from build123d import *

# Parameters (mm, degrees)
SKETCH1_W           = 37
SKETCH1_H           = 22
BOSS_EXTRUDE1_DEPTH = 10
SKETCH3_W           = 37
SKETCH3_H           = 22
BOSS_EXTRUDE2_DEPTH = 9
SKETCH5_W           = 5
SKETCH5_H           = 3
BOSS_EXTRUDE3_DEPTH = 5
SKETCH6_R           = 1.5
CUT_EXTRUDE1_DEPTH  = 5
FILLET1_R           = 0.4
FILLET2_R           = 4
SKETCH7_R           = 3
CUT_EXTRUDE2_DEPTH  = 44.023249529
SKETCH8_R           = 1.5
CUT_EXTRUDE4_DEPTH  = 44.023249529
SKETCH10_R          = 2
CUT_EXTRUDE5_DEPTH  = 2
BOSS_EXTRUDE4_DEPTH = 11
CUT_EXTRUDE6_DEPTH  = 11
SKETCH13_W          = 3
SKETCH13_H          = 5
BOSS_EXTRUDE5_DEPTH = 2
CUT_EXTRUDE7_DEPTH  = 51.955863254


with BuildPart() as part:
    # Sketch1 → Boss-Extrude1 (new body)
    with BuildSketch(Plane(origin=(0, 0, 0), x_dir=(1, 0, 0), z_dir=(0, 1, 0))):
        with Locations((-18.5, 0)):
            Rectangle(SKETCH1_W, SKETCH1_H)
    extrude(amount=BOSS_EXTRUDE1_DEPTH)

    # Sketch3 → Boss-Extrude2 (add)
    with BuildSketch(Plane.XZ):
        with Locations((-18.5, 0)):
            Rectangle(SKETCH3_W, SKETCH3_H)
    extrude(amount=BOSS_EXTRUDE2_DEPTH)

    # Sketch5 → Boss-Extrude3 (add)
    with BuildSketch(Plane(origin=(0, 0, 0), x_dir=(0, 0, -1), z_dir=(1, 0, 0))):
        Rectangle(SKETCH5_W, SKETCH5_H)
    extrude(amount=BOSS_EXTRUDE3_DEPTH)

    # Sketch6 → Cut-Extrude1 (cut)
    with BuildSketch(Plane(origin=(0, 1.5, 0), x_dir=(1, 0, 0), z_dir=(0, 1, 0))):
        with Locations(Location((2.5, 0, 0), (0, 0, 270))):
            Circle(SKETCH6_R)
    extrude(amount=-CUT_EXTRUDE1_DEPTH, mode=Mode.SUBTRACT)

    # Fillet1
    fillet1_edges = [part.edges().sort_by_distance(p)[0] for p in [
        (5, 0, -2.5),
        (5, 0, 2.5),
    ]]
    fillet(fillet1_edges, radius=FILLET1_R)

    # Fillet2
    fillet2_edges = [part.edges().sort_by_distance(p)[0] for p in [
        (0, 0.5, 11),
        (0, 0.5, -11),
    ]]
    fillet(fillet2_edges, radius=FILLET2_R)

    # Sketch7 → Cut-Extrude2 (cut, through all)
    with BuildSketch(Plane(origin=(0, 10, 0), x_dir=(1, 0, 0), z_dir=(0, 1, 0))):
        with Locations(Location((-11, 0, 0), (0, 0, 270))):
            Circle(SKETCH7_R)
    extrude(amount=-CUT_EXTRUDE2_DEPTH, mode=Mode.SUBTRACT)

    # Sketch8 → Cut-Extrude4 (cut, through all)
    with BuildSketch(Plane(origin=(0, 10, 0), x_dir=(1, 0, 0), z_dir=(0, 1, 0))):
        with Locations(Location((-32, 8.7, 0), (0, 0, 270))):
            Circle(SKETCH8_R)
        with Locations(Location((-32, -8.7, 0), (0, 0, 270))):
            Circle(SKETCH8_R)
    extrude(amount=-CUT_EXTRUDE4_DEPTH, mode=Mode.SUBTRACT)

    # Sketch10 → Cut-Extrude5 (cut)
    with BuildSketch(Plane(origin=(0, 10, 0), x_dir=(1, 0, 0), z_dir=(0, 1, 0))):
        with Locations(Location((-34.5, 6, 0), (0, 0, 270))):
            Circle(SKETCH10_R)
        with Locations(Location((-34.5, -6, 0), (0, 0, 270))):
            Circle(SKETCH10_R)
    extrude(amount=-CUT_EXTRUDE5_DEPTH, mode=Mode.SUBTRACT)

    # Sketch11 → Boss-Extrude4 (add)
    with BuildSketch(Plane.ZY.offset(37)):
        with BuildLine():
            Line((-6.164414003, 8.5), (6.164414003, 8.5))
            ThreePointArc((6.164414003, 8.5), (10.5, 0), (6.164414003, -8.5))
            Line((6.164414003, -8.5), (-6.164414003, -8.5))
            ThreePointArc((-6.164414003, -8.5), (-10.5, 0), (-6.164414003, 8.5))
        make_face()
    extrude(amount=BOSS_EXTRUDE4_DEPTH)

    # Sketch12 → Cut-Extrude6 (cut)
    with BuildSketch(Plane.ZY.offset(48)):
        with BuildLine():
            Line((-5.830951895, -7.5), (5.830951895, -7.5))
            ThreePointArc((5.830951895, -7.5), (9.5, 0), (5.830951895, 7.5))
            Line((5.830951895, 7.5), (-5.830951895, 7.5))
            ThreePointArc((-5.830951895, 7.5), (-9.5, 0), (-5.830951895, -7.5))
        make_face()
    extrude(amount=-CUT_EXTRUDE6_DEPTH, mode=Mode.SUBTRACT)

    # Sketch13 → Boss-Extrude5 (add)
    with BuildSketch(Plane(origin=(0, 8.5, 0), x_dir=(1, 0, 0), z_dir=(0, 1, 0))):
        with Locations((-43.5, 0)):
            Rectangle(SKETCH13_W, SKETCH13_H)
    boss_extrude5 = extrude(amount=BOSS_EXTRUDE5_DEPTH)

    # Sketch14 → Cut-Extrude7 (cut, through all)
    with BuildSketch(Plane.XY.offset(2.5)):
        Polygon((-44.5, 9.5), (-44, 10.5), (-45, 10.5), (-45, 9.5), align=None)
        Polygon((-45, 8.5), (-44.5, 9.5), (-45, 9.5), align=None)
        Polygon((-42, 9.5), (-43.5, 9.5), (-44, 8.5), (-42, 8.5), align=None)
    cut_extrude7 = extrude(amount=-CUT_EXTRUDE7_DEPTH, mode=Mode.SUBTRACT)

    # Mirror2: Boss-Extrude5 across plane
    add(boss_extrude5.mirror(Plane.ZX))

    # Mirror3: Cut-Extrude7 across plane
    add(cut_extrude7.mirror(Plane.ZX), mode=Mode.SUBTRACT)


solid = part.part
For this review, take the finished solid that the model builds, in its own axes (mm). A direction names the side the tool comes from. Round coordinates to 2 decimals unless told otherwise and drop trailing zeros. Order: outer loops, then holes, each group sorted by start corner. A loop starts at its lowest first (then second) coordinate and runs counter-clockwise, first axis right, second up. Notation, with made-up numbers: M -30,41.25 L 27,41.25 A36 cw 27,79.25 Z; hole C 62.5,68 d3. An arc over 180 degrees is marked long. Use a Markdown table: item, result. Add a question column.
Item 1: Add section B-B, the plane z = -8.7. Give the boundary of the cut face in (x, y).
Item 2: Mouldability with a two-part tool opening along Z and no side actions: class faces 1 (the flat face through (-19, -9, 0)), 2 (the flat face through (-44, -10, 2.5)), 3 (the cylindrical face through (-42.6, -0.1, 9.5)) as released by +Z, released by -Z, zero draft, split by the parting line, or undercut.
Item 3: Tool access review of faces 4 (the cylindrical face through (-36.452, 9.014, -6.434)), 5 (the flat face through (-42, -10, 0)), 6 (the flat face through (-44, -10, -2.5)): name each direction out of +Z, -Z, +X, -X, +Y, -Y from which nothing blocks a thin tool from reaching the whole face with its end or side.
Item 4: Add section A-A, the plane x = -32. Give the boundary of the cut face in (y, z), then the cut area to 3 significant figures.
Item 5: Add section C-C, the plane y = -4.5. Give the boundary of the cut face in (x, z), then the cut area to 3 significant figures.
Item 6: Add section D-D, the plane z = 0. State how many separate pieces and enclosed holes the cut face has, then the cut area to 4 significant figures.
Item 7: Insertion check: pin 1 (0.6 mm diameter, centred on x = -43.5, y = -9.5, fed in from -Z); pin 2 (1.2 mm diameter, centred on x = -35, z = -5.5, fed in from +Y); pin 3 (11 mm diameter, centred on x = -10, z = -3, fed in from -Y); pin 4 (12 mm diameter, centred on x = -40, z = 0.5, fed in from +Y). Each pin has a flat end and moves straight along its axis. Give the tip position at first contact, or say it passes through.
Item 8: To check wall thickness, follow line 1 along X through (y, z) = (0, 0); line 2 along X through (y, z) = (-1.75, 0.25); line 3 along Y through (x, z) = (-25, 8.25). State the ranges of each line that lie inside material, in increasing order.
Geometry results:
| question | item | result |
|---|---|---|
| 1 | outline | M -48,-5.88 L -37,-5.88 L -37,-9 L -33.5,-9 L -33.5,10 L -37,10 L -37,5.88 L -48,5.88 L -48,3.82 L -37,3.82 L -37,-3.82 L -48,-3.82 Z; M -30.5,-9 L -0.38,-9 L -0.38,10 L -30.5,10 Z |
| 2 | face 1 | zero draft |
| 2 | face 2 | released by +Z |
| 2 | face 3 | undercut |
| 3 | face 4 | +Y |
| 3 | face 5 | +Z, -Z, +X, -Y |
| 3 | face 6 | -Z, -X, -Y |
| 4 | outline | M -9,-11 L 10,-11 L 10,-10.2 L -9,-10.2 Z; M -9,-7.2 L 10,-7.2 L 10,7.2 L -9,7.2 Z; M -9,10.2 L 10,10.2 L 10,11 L -9,11 Z |
| 4 | area | 304 mm² |
| 5 | outline | M -48,-9.49 L -37,-9.49 L -37,-11 L -4,-11 A4 ccw 0,-7 L 0,7 A4 ccw -4,11 L -37,11 L -37,9.49 L -48,9.49 L -48,8.37 L -37,8.37 L -37,-8.37 L -48,-8.37 Z; hole C -32,-8.7 d3; hole C -32,8.7 d3; hole C -11,0 d6 |
| 5 | area | 789 mm² |
| 6 | separate pieces | 3 |
| 6 | enclosed holes | 0 |
| 6 | area | 623.5 mm² |
| 7 | pin 1 | stops at z = -2.5 |
| 7 | pin 2 | stops at y = 8 |
| 7 | pin 3 | stops at y = -9 |
| 7 | pin 4 | stops at y = 10.5 |
| 8 | line 1 | x = -37 to -14, -8 to 1, 4 to 5 |
| 8 | line 2 | x = -37 to -13.99, -8.01 to 0 |
| 8 | line 3 | y = -9 to 10 |
